from build123d import *
from build123d.topology import SkipClean

# Parameters (mm, degrees)
BOSS_EXTRUDE1_DEPTH = 0.5
SKETCH5_R           = 5
CUT_EXTRUDE1_DEPTH  = 27


with BuildPart() as part:
    # Sketch2 → Boss-Extrude1 (new body)
    with BuildSketch(Plane.XY):
        with BuildLine():
            Line((-17.5, -0.25), (-13.5, -0.25))
            ThreePointArc((-13.5, -0.25), (-12.616116524, 0.116116524), (-12.25, 1))
            Line((-12.25, 1), (-12.25, 7))
            ThreePointArc((-12.25, 7), (-11, 8.25), (-9.75, 7))
            Line((-9.75, 7), (-9.75, 0))
            Line((-9.75, 0), (-9.75, -7))
            ThreePointArc((-9.75, -7), (-8, -8.75), (-6.25, -7))
            Line((-6.25, -7), (-6.25, 0))
            Line((-6.25, 0), (-6.25, 7))
            ThreePointArc((-6.25, 7), (-5, 8.25), (-3.75, 7))
            Line((-3.75, 7), (-3.75, 0))
            Line((-3.75, 0), (-3.75, -7))
            ThreePointArc((-3.75, -7), (-2, -8.75), (-0.25, -7))
            Line((-0.25, -7), (-0.25, 0))
            Line((-0.25, 0), (-0.25, 7))
            ThreePointArc((-0.25, 7), (1, 8.25), (2.25, 7))
            Line((2.25, 7), (2.25, 0))
            Line((2.25, 0), (2.25, -7))
            ThreePointArc((2.25, -7), (4, -8.75), (5.75, -7))
            Line((5.75, -7), (5.75, -1))
            ThreePointArc((5.75, -1), (5.969669914, -0.469669914), (6.5, -0.25))
            Line((6.5, -0.25), (10.5, -0.25))
            ThreePointArc((10.5, -0.25), (10.75, 0), (10.5, 0.25))
            Line((10.5, 0.25), (6.5, 0.25))
            ThreePointArc((6.5, 0.25), (5.616116524, -0.116116524), (5.25, -1))
            Line((5.25, -1), (5.25, -7))
            ThreePointArc((5.25, -7), (4, -8.25), (2.75, -7))
            Line((2.75, -7), (2.75, 0))
            Line((2.75, 0), (2.75, 7))
            ThreePointArc((2.75, 7), (1, 8.75), (-0.75, 7))
            Line((-0.75, 7), (-0.75, 0))
            Line((-0.75, 0), (-0.75, -7))
            ThreePointArc((-0.75, -7), (-2, -8.25), (-3.25, -7))
            Line((-3.25, -7), (-3.25, 0))
            Line((-3.25, 0), (-3.25, 7))
            ThreePointArc((-3.25, 7), (-5, 8.75), (-6.75, 7))
            Line((-6.75, 7), (-6.75, 0))
            Line((-6.75, 0), (-6.75, -7))
            ThreePointArc((-6.75, -7), (-8, -8.25), (-9.25, -7))
            Line((-9.25, -7), (-9.25, 0))
            Line((-9.25, 0), (-9.25, 7))
            ThreePointArc((-9.25, 7), (-11, 8.75), (-12.75, 7))
            Line((-12.75, 7), (-12.75, 1))
            ThreePointArc((-12.75, 1), (-12.969669914, 0.469669914), (-13.5, 0.25))
            Line((-13.5, 0.25), (-17.5, 0.25))
            ThreePointArc((-17.5, 0.25), (-17.75, 0), (-17.5, -0.25))
        make_face()
    extrude(amount=BOSS_EXTRUDE1_DEPTH)

    # Sketch3 → Revolve1 (revolve)
    with SkipClean():  # the faces are left unmerged after this step: merging them gives an invalid solid
        with BuildSketch(Plane(origin=(0, 0, 0), x_dir=(-1, 0, 0), z_dir=(0, -1, 0)), mode=Mode.PRIVATE) as revolve1_sk:
            Polygon((17.5, -0.5), (22.5, -0.5), (23.5, 3.5), (23.5, 29.5), (17.5, 29.5), align=None)
        revolve(revolve1_sk.sketch.rotate(Axis((-17.5, 0, 0.5), (0, 0, -1)), 157.945831956), axis=Axis((-17.5, 0, 0.5), (0, 0, -1)))

    # Sketch4 → Revolve2 (revolve)
    with SkipClean():  # the faces are left unmerged after this step: merging them gives an invalid solid
        with BuildSketch(Plane(origin=(0, 0, 0), x_dir=(-1, 0, 0), z_dir=(0, -1, 0)), mode=Mode.PRIVATE) as revolve2_sk:
            Polygon((-10.5, -0.5), (-15.5, -0.5), (-16.5, 3.5), (-16.5, 29.5), (-10.5, 29.5), align=None)
        revolve(revolve2_sk.sketch.rotate(Axis((10.5, 0, 0.5), (0, 0, -1)), 177.22310556), axis=Axis((10.5, 0, 0.5), (0, 0, -1)))

    # Sketch5 → Cut-Extrude1 (cut)
    with SkipClean():  # the faces are left unmerged after this step: merging them gives an invalid solid
        with BuildSketch(Plane(origin=(0, 0, -29.5), x_dir=(-1, 0, 0), z_dir=(0, 0, -1))):
            with Locations((-10.5, 0)):
                Circle(SKETCH5_R)
            with Locations((17.5, 0)):
                Circle(SKETCH5_R)
        extrude(amount=-CUT_EXTRUDE1_DEPTH, mode=Mode.SUBTRACT)


solid = part.part
Model file for the job. Use its own axes, mm. A direction names the side the tool comes from. Round coordinates to 2 decimals unless told otherwise and drop trailing zeros. Loops run counter-clockwise (first coordinate to the right, second up) from the corner with the lowest first, then second, coordinate; pieces in that order, holes last.
1. Band-saw the part on C-C, the plane y = 3.75. Count the separate pieces of the cut face and the enclosed holes in it, and give its area (3 significant figures).
Check values:
separate pieces: 8
enclosed holes: 0
area: 196 mm2
2. Drop flat-ended pins along their axis: P1, Ø0.6, axis at y = -3.5, z = 0, coming from the +X side; P2, Ø5, axis at x = -4.5, y = -2, coming from the -Z side; P3, Ø2, axis at y = -2.5, z = -20, coming from the -X side. Give the stop position or say it passes through.
Check values:
P1: stops at x = 14.52
P2: stops at z = 0
P3: stops at x = -23.31
3. Wall check: probe 1 along Y at (x, z) = (10.5, -20); probe 2 along X at (y, z) = (-4, -7.5); probe 3 along X at (y, z) = (-0.75, -12.5). Give the ranges that are in metal, low to high.
Check values:
probe 1: y = -6 to -5, 5 to 6
probe 2: x = -21.97 to -20.5, -14.5 to -13.03, 6.03 to 7.5, 13.5 to 14.97
probe 3: x = -23.45 to -22.44, -12.56 to -11.55, 4.55 to 5.56, 15.44 to 16.45
4. Tool access for faces 5 (the cylindrical face through (0.97, 8.25, 0.25)), 6 (the cylindrical face through (-12.505, 0.22, -16.189)): list every direction of +Z, -Z, +X, -X, +Y, -Y with a clear straight run to the whole face (end or side of a thin tool).
Check values:
face 5: +Z, -Z, -Y
face 6: -Z
5. Mould opens along Y. For faces 1 (the cylindrical face through (3.96, -8.75, 0.25)), 2 (the flat face through (13, 5, -29.5)), 3 (the cylindrical face through (-1.97, -8.25, 0.25)), 4 (the cylindrical face through (5.73, 1.5, -16.19)) say: +Y half, -Y half, draft (parallel to the pull), parting line (faces both ways), or undercut.
Check values:
face 1: -Y half
face 2: draft
face 3: +Y half
face 4: undercut
6. Band-saw the part on A-A, the plane z = -14.5. List the corners of the cut face in (x, y), and give its area (3 significant figures).
Check values:
outline: circle Ø12 at (-17.5, 0); circle Ø12 at (10.5, 0); hole circle Ø10 at (-17.5, 0); hole circle Ø10 at (10.5, 0)
area: 69.1 mm2
7. Band-saw the part on D-D, the plane z = -2. List the corners of the cut face in (x, y) (3 decimals), and give its area (3 significant figures).
Check values:
outline: circle Ø11.25 at (-17.5, 0); circle Ø11.25 at (10.5, 0)
area: 199 mm2
8. Band-saw the part on B-B, the plane x = -2. List the corners of the cut face in (y, z).
Check values:
outline: (-8.75, 0) - (-8.25, 0) - (-8.25, 0.5) - (-8.75, 0.5) - close
